CAD build for the part. Positions are in the model's coordinates, mm. A direction names the side the tool comes from. Give positions to 0.01 mm unless a question says otherwise; leave off trailing zeros. Loops run counter-clockwise (first coordinate to the right, second up) from the corner with the lowest first, then second, coordinate; pieces in that order, holes last.
```python
from build123d import *

# Parameters (mm, degrees)
SKETCH1_W           = 150.9
SKETCH1_H           = 90
SKETCH1_R           = 1.5
SKETCH1_W_2         = 10
SKETCH1_H_2         = 3
SKETCH1_W_3         = 3
SKETCH1_H_3         = 10
BOSS_EXTRUDE1_DEPTH = 3


with BuildPart() as part:
    # Sketch1 → Boss-Extrude1 (new body)
    with BuildSketch(Plane(origin=(0, 0, 0), x_dir=(1, 0, 0), z_dir=(0, 1, 0))):
        with Locations((-75.45, 45)):
            Rectangle(SKETCH1_W, SKETCH1_H)
        with Locations(Location((-57, 84.5, 0), (0, 0, 270))):
            Circle(SKETCH1_R, mode=Mode.SUBTRACT)
        with Locations(Location((-107, 84.5, 0), (0, 0, 270))):
            Circle(SKETCH1_R, mode=Mode.SUBTRACT)
        with Locations(Location((-107, 5.5, 0), (0, 0, 90))):
            Circle(SKETCH1_R, mode=Mode.SUBTRACT)
        with Locations(Location((-57, 5.5, 0), (0, 0, 90))):
            Circle(SKETCH1_R, mode=Mode.SUBTRACT)
        with Locations(Location((-5.5, 45, 0), (0, 0, 270))):
            Circle(SKETCH1_R, mode=Mode.SUBTRACT)
        with Locations((-32, 84.5)):
            Rectangle(SKETCH1_W_2, SKETCH1_H_2, mode=Mode.SUBTRACT)
        with Locations((-82, 84.5)):
            Rectangle(SKETCH1_W_2, SKETCH1_H_2, mode=Mode.SUBTRACT)
        with Locations((-132, 84.5)):
            Rectangle(SKETCH1_W_2, SKETCH1_H_2, mode=Mode.SUBTRACT)
        with Locations((-132, 5.5)):
            Rectangle(SKETCH1_W_2, SKETCH1_H_2, mode=Mode.SUBTRACT)
        with Locations((-82, 5.5)):
            Rectangle(SKETCH1_W_2, SKETCH1_H_2, mode=Mode.SUBTRACT)
        with Locations((-32, 5.5)):
            Rectangle(SKETCH1_W_2, SKETCH1_H_2, mode=Mode.SUBTRACT)
        with Locations((-5.5, 67.5)):
            Rectangle(SKETCH1_W_3, SKETCH1_H_3, mode=Mode.SUBTRACT)
        with Locations((-5.5, 22.5)):
            Rectangle(SKETCH1_W_3, SKETCH1_H_3, mode=Mode.SUBTRACT)
    extrude(amount=BOSS_EXTRUDE1_DEPTH)


solid = part.part
```
1. Probe line 1 along X through (y, z) = (1.2, -5.5); line 2 along Z through (x, y) = (-129, 2.75); line 3 along X through (y, z) = (1, -69). List the from-to ranges inside material, lowest first.
Responses:
line 1: x = -150.9 to -137, -127 to -108.5, -105.5 to -87, -77 to -58.5, -55.5 to -37, -27 to 0
line 2: z = -90 to -86, -83 to -7, -4 to 0
line 3: x = -150.9 to -7, -4 to 0
2. Tool access for faces 4 (the face through (-77, 3, -46)), 5 (the face through (-4, 1, -22)): list every direction of +Z, -Z, +X, -X, +Y, -Y with a clear straight run to the whole face (end or side of a thin tool).
Responses:
face 4: +Z, -Z, +X, -X, +Y
face 5: +Y, -Y
3. Saw through at B-B, the plane x = -5.5. List the corners of the cut face in (y, z), and give its area (3 significant figures).
Responses:
outline: (0, -90) - (3, -90) - (3, -72.5) - (0, -72.5) - close; (0, -62.5) - (3, -62.5) - (3, -46.5) - (0, -46.5) - close; (0, -43.5) - (3, -43.5) - (3, -27.5) - (0, -27.5) - close; (0, -17.5) - (3, -17.5) - (3, 0) - (0, 0) - close
area: 201 mm2
4. Saw through at A-A, the plane z = -84.5. List the corners of the cut face in (x, y).
Responses:
outline: (-150.9, 0) - (-137, 0) - (-137, 3) - (-150.9, 3) - close; (-127, 0) - (-108.5, 0) - (-108.5, 3) - (-127, 3) - close; (-105.5, 0) - (-87, 0) - (-87, 3) - (-105.5, 3) - close; (-77, 0) - (-58.5, 0) - (-58.5, 3) - (-77, 3) - close; (-55.5, 0) - (-37, 0) - (-37, 3) - (-55.5, 3) - close; (-27, 0) - (0, 0) - (0, 3) - (-27, 3) - close
5. Saw through at D-D, the plane x = -107. List the corners of the cut face in (y, z), and give its area (3 significant figures).
Responses:
outline: (0, -90) - (3, -90) - (3, -86) - (0, -86) - close; (0, -83) - (3, -83) - (3, -7) - (0, -7) - close; (0, -4) - (3, -4) - (3, 0) - (0, 0) - close
area: 252 mm2
6. Pull direction X, two halves, no side cores. Call faces 1 (the face through (-132, 1, -83)), 2 (the face through (-132, 1, -4)), 3 (the face through (-77, 1, -90)): released by +X, released by -X, zero draft, split by the parting line, or undercut.
Responses:
face 1: undercut
face 2: undercut
face 3: zero draft
7. Saw through at C-C, the plane z = -45. List the corners of the cut face in (x, y), and give its area (3 significant figures).
Responses:
outline: (-150.9, 0) - (-7, 0) - (-7, 3) - (-150.9, 3) - close; (-4, 0) - (0, 0) - (0, 3) - (-4, 3) - close
area: 444 mm2
8. Drop a flat-ended pin along its axis: pin 1 (1.5 mm diameter, centred on x = -130.5, y = 1, fed in from +Z). Give the stop position or say it passes through.
Responses:
pin 1: stops at z = 0
